from build123d import *

# Parameters (mm, degrees)
SKETCH1_W           = 18.5
SKETCH1_H           = 4
BOSS_EXTRUDE1_DEPTH = 0.75
SKETCH2_W           = 8
SKETCH2_H           = 4.2
BOSS_EXTRUDE2_DEPTH = 0.75


with BuildPart() as part:
    # Sketch1 → Boss-Extrude1 (new body)
    with BuildSketch(Plane.XY):
        Rectangle(SKETCH1_W, SKETCH1_H)
    boss_extrude1 = extrude(amount=BOSS_EXTRUDE1_DEPTH)

    # Sketch2 → Boss-Extrude2 (add)
    with BuildSketch(Plane.XY):
        with Locations((0, -4.1)):
            Rectangle(SKETCH2_W, SKETCH2_H)
    boss_extrude2 = extrude(amount=BOSS_EXTRUDE2_DEPTH)

    # Mirror1: Boss-Extrude1, Boss-Extrude2 across plane
    add(boss_extrude1.mirror(Plane.XY))
    add(boss_extrude2.mirror(Plane.XY))


solid = part.part
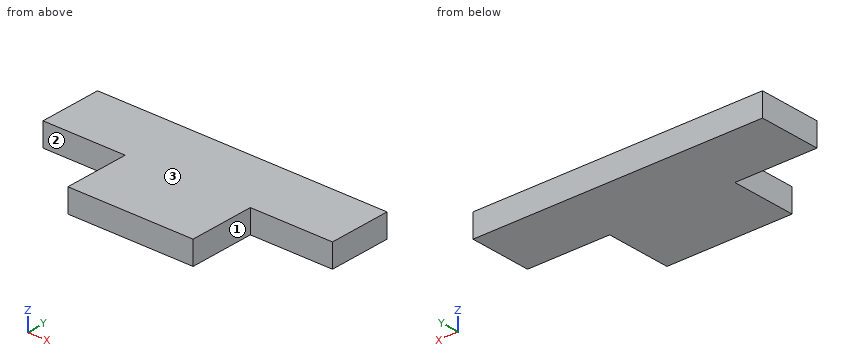
Design review of the part built by this model. Coordinates are the model's own, in mm. Face numbers are marked on the shaded views. A direction names the side the tool comes from. Give positions to 0.01 mm unless a question says otherwise; leave off trailing zeros. Write each loop counter-clockwise with the first axis right and the second up, starting at its lowest first coordinate (ties: lowest second). Pieces come first, ordered by that corner, then holes. Notation, with made-up numbers: M 64,71.5 L 74,71.5 A11 ccw 74,86.5 Z; hole C 29.5,20 d8. An arc over 180 degrees is marked long. Return JSON: item names as keys, results as strings. Group by question number.
Item 1: Take a section at A-A (z = 0.15). Give the boundary of the cut face in (x, y), plus the area to 3 significant figures.
Item 2: Take a section at B-B (y = -3.75). Give the boundary of the cut face in (x, z).
Item 3: Wall thickness on line 1 along X through (y, z) = (-3.75, 0.2); line 2 along Y through (x, z) = (7.25, -0.35): over which ranges is each line inside the solid? List them lowest first.
Item 4: Take a section at C-C (x = 6.25). Give the boundary of the cut face in (y, z), plus the area to 3 significant figures.
Item 5: Tool access review of the marked faces 1, 2 and 3: name each direction out of +Z, -Z, +X, -X, +Y, -Y from which nothing blocks a thin tool from reaching the whole face with its end or side.
Return value:
{
 "1": {"outline": "M -9.25,-2 L -4,-2 L -4,-6.2 L 4,-6.2 L 4,-2 L 9.25,-2 L 9.25,2 L -9.25,2 Z", "area": "108 mm2"},
 "2": {"outline": "M -4,-0.75 L 4,-0.75 L 4,0.75 L -4,0.75 Z"},
 "3": {"line 1": "x = -4 to 4", "line 2": "y = -2 to 2"},
 "4": {"outline": "M -2,-0.75 L 2,-0.75 L 2,0.75 L -2,0.75 Z", "area": "6.00 mm2"},
 "5": {"face 1": "+Z, -Z, +X, -Y", "face 2": "+Z, -Z, -X, -Y", "face 3": "+Z, +X, -X, +Y, -Y"}
}
